Geometry check sheet. Reference: the model listing, model coordinates, mm. Round coordinates to 2 decimals unless told otherwise and drop trailing zeros. Order: outer loops, then holes, each group sorted by start corner. A loop starts at its lowest first (then second) coordinate and runs counter-clockwise, first axis right, second up. Notation, with made-up numbers: (56.5, 86) - (92.5, 86) arc R19 cw to (92.5, 106) - close; hole circle Ø8 at (45.25, 2.5). An arc over 180 degrees is marked (long way). Return JSON: item names as keys, results as strings. Group by question number.
Q1. Sectioned sample at D-D, the plane x = -55.5. Record the cut outline in (y, z).
Q2. Gauge pin test, flat end, axial feed: pin 1 Ø1 at (x, z) = (31, 5) entering from -Y. Record the tip position at first contact, or that the pin passes through.
Q3. Sectioned sample at A-A, the plane y = -127. Record the cut outline in (x, z) (3 decimals).
Q4. Material ranges on line 1 along X through (y, z) = (-127, 1.5) (3 decimals); line 2 along X through (y, z) = (-12, 3); line 3 along X through (y, z) = (17.5, 0.5), recorded low to high.
Q5. Sectioned sample at B-B, the plane y = -59. Record the cut outline in (x, z), then the cut area to 3 significant figures.
Q6. Sectioned sample at C-C, the plane z = 3.75. Record the cut outline in (x, y) (3 decimals).
Autodesk Inventor part; units mm, degrees
ref_plane "YZ Plane" through (0, 0, 0) normal (1, 0, 0) x (0, 1, 0)
ref_plane "XZ Plane" through (0, 0, 0) normal (0, 1, 0) x (-1, 0, 0)
ref_plane "XY Plane" through (0, 0, 0) normal (0, 0, 1) x (1, 0, 0)
sketch "Sketch1" plane through (0, 0, 0) normal (0, 0, 1) x (1, 0, 0)
  line L0 (-254, 254) -> (254, 254)
  line L1 (254, 254) -> (254, -254)
  line L2 (-254, -254) -> (-254, 254)
  line L3 (-254, 254) -> (254, -254) construction
  line L4 (254, 254) -> (-254, -254) construction
  line L5 (-254, -254) -> (-152.4, -152.4)
  line L6 (-152.4, -152.4) -> (-152.4, 152.4)
  line L7 (-152.4, 152.4) -> (152.4, 152.4)
  line L8 (152.4, 152.4) -> (152.4, -152.4)
  line L9 (254, -254) -> (152.4, -152.4)
  point P0 (0, 0)
  dimension "d2" = 101.6
  dimension "d3" = 101.6
  dimension "d23" = 304.8
extrude "Extrusion1" add sketch "Sketch1" along normal blind 6.35
sketch "Sketch2" plane through (0, 0, 6.35) normal (0, 0, 1) x (1, 0, 0)
  line L0 (-152.4, -152.4) -> (-152.4, 152.4)
  line L1 (152.4, 152.4) -> (152.4, -152.4)
  circle A0 centre (-180.975, -127) radius 50.8 construction
  line L2 (-254, -254) -> (-152.4, -152.4) construction
  point P0 (0, 0)
  point P1 (-190.5, 25.2039)
  point P2 (190.5, 25.2039)
  point P3 (180.975, -127)
  dimension "d6" = 28.575
  dimension "d7" = 38.1
  dimension "d8" = 38.1
  dimension "d9" = 28.575
  dimension "d18" = 152.5016
  dimension "d20" = 152.5016
  dimension "d21" = 101.6
  dimension "d25" = 127
hole "Hole1" at (-180.975, -127, 6.35) at (-190.5, 25.2039, 6.35) at (190.5, 25.2039, 6.35) at (180.975, -127, 6.35) direction (0, 0, -1) diameter 27.94 end through all
fillet "Fillet1" radius 13.97 2 edges at (-152.4, 152.4, 3.175) (152.4, 152.4, 3.175)
fillet "Fillet2" radius 6.35 2 edges at (-254, -254, 3.175) (254, -254, 3.175)
properties part number "AI1-001" material "Aluminum 6061"
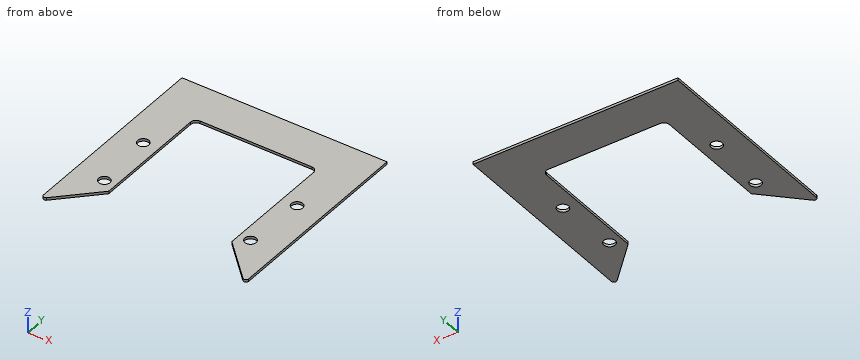
Reply:
{
 "1": {"outline": "(152.4, 0) - (254, 0) - (254, 6.35) - (152.4, 6.35) - close"},
 "2": {"pin 1": "y = 152.4"},
 "3": {"outline": "(-254, 0) - (-194.945, 0) - (-194.945, 6.35) - (-254, 6.35) - close; (-167.005, 0) - (-152.4, 0) - (-152.4, 6.35) - (-167.005, 6.35) - close; (152.4, 0) - (167.005, 0) - (167.005, 6.35) - (152.4, 6.35) - close; (194.945, 0) - (254, 0) - (254, 6.35) - (194.945, 6.35) - close"},
 "4": {"line 1": "-254 to -194.945, -167.005 to -152.4, 152.4 to 167.005, 194.945 to 254", "line 2": "-254 to -152.4, 152.4 to 254", "line 3": "-254 to -202.15, -178.85 to -152.4, 152.4 to 178.85, 202.15 to 254"},
 "5": {"outline": "(-254, 0) - (-152.4, 0) - (-152.4, 6.35) - (-254, 6.35) - close; (152.4, 0) - (254, 0) - (254, 6.35) - (152.4, 6.35) - close", "area": "1,290 mm^2"},
 "6": {"outline": "(-254, -238.67) arc R6.35 ccw to (-243.16, -243.16) - (-152.4, -152.4) - (-152.4, 138.43) arc R13.97 cw to (-138.43, 152.4) - (138.43, 152.4) arc R13.97 cw to (152.4, 138.43) - (152.4, -152.4) - (243.16, -243.16) arc R6.35 ccw to (254, -238.67) - (254, 254) - (-254, 254) - close; hole circle Ø27.94 at (-190.5, 25.204); hole circle Ø27.94 at (-180.975, -127); hole circle Ø27.94 at (180.975, -127); hole circle Ø27.94 at (190.5, 25.204)"}
}
